from build123d import *

# Parameters (mm, degrees)
EXTRUDE_1_DEPTH     = 4
SKETCH_2_R          = 1.5
CUT_EXTRUDE_1_DEPTH = 53.719070053
CUT_EXTRUDE_3_DEPTH = 2.4
EXTRUDE_2_DEPTH     = 2
FILLET_3_R          = 2
CHAMFER_1_SIZE      = 2


with BuildPart() as part:
    # Эскиз1 → Бобышка-Вытянуть1 (new body)
    with BuildSketch(Plane(origin=(0, 0, 0), x_dir=(0, 0, -1), z_dir=(1, 0, 0))):
        Polygon((-49.583333333, 6.541666667), (-49.583333333, -17.458333333), (-5.983333333, -17.458333333), (-5.983333333, 6.541666667), (-14.983333333, 6.541666667), (-14.983333333, -8.458333333), (-40.583333333, -8.458333333), (-40.583333333, 6.541666667), align=None)
    extrude(amount=EXTRUDE_1_DEPTH)

    # Эскиз2 → Вырез-Вытянуть1 (cut, through all)
    with BuildSketch(Plane.ZY):
        with Locations((10.483333333, 2.190961295)):
            Circle(SKETCH_2_R)
        with Locations((45.083333333, 2.190961295)):
            Circle(SKETCH_2_R)
    extrude(amount=-CUT_EXTRUDE_1_DEPTH, mode=Mode.SUBTRACT)

    # Эскиз4 → Вырез-Вытянуть3 (cut)
    with BuildSketch(Plane.ZY):
        Polygon((10.483333333, 5.337520262), (7.758333333, 3.764240779), (7.758333333, 0.617681812), (10.483333333, -0.955597672), (13.208333333, 0.617681812), (13.208333333, 3.764240779), align=None)
        Polygon((45.083333333, 5.337520262), (42.358333333, 3.764240779), (42.358333333, 0.617681812), (45.083333333, -0.955597672), (47.808333333, 0.617681812), (47.808333333, 3.764240779), align=None)
    extrude(amount=-CUT_EXTRUDE_3_DEPTH, mode=Mode.SUBTRACT)

    # Эскиз6 → Бобышка-Вытянуть2 (add)
    with BuildSketch(Plane.ZY):
        Polygon((5.983333333, -6.458333333), (14.983333333, -6.458333333), (14.983333333, -8.458333333), (40.583333333, -8.458333333), (40.583333333, -6.458333333), (49.583333333, -6.458333333), (49.583333333, -17.458333333), (5.983333333, -17.458333333), align=None)
    extrude(amount=EXTRUDE_2_DEPTH)

    # Скругление3
    fillet_3_edges = [part.edges().sort_by_distance(p)[0] for p in [
        (2, 6.541666667, 40.583333333),
        (2, 6.541666667, 14.983333333),
        (2, 6.541666667, 5.983333333),
        (1, -17.458333333, 5.983333333),
        (1, -17.458333333, 49.583333333),
        (2, 6.541666667, 49.583333333),
    ]]
    fillet(fillet_3_edges, radius=FILLET_3_R)

    # Фаска1
    chamfer_1_edges = [part.edges().sort_by_distance(p)[0] for p in [
        (-2, -6.458333333, 10.483333333),
        (-2, -6.458333333, 45.083333333),
    ]]
    chamfer(chamfer_1_edges, length=CHAMFER_1_SIZE - 0.0001)  # a hair under: the kernel refuses the full size


solid = part.part
For this review, take the finished solid that the model builds, in its own axes (mm). A direction names the side the tool comes from. Give positions to 0.01 mm unless a question says otherwise; leave off trailing zeros. Order: outer loops, then holes, each group sorted by start corner. A loop starts at its lowest first (then second) coordinate and runs counter-clockwise, first axis right, second up. Notation, with made-up numbers: (88, 79) - (100, 79) arc R32 ccw to (100, 118) - close; hole circle Ø5 at (-34, 39.5). An arc over 180 degrees is marked (long way). Answer as a JSON object with one key per item and string values. Group by question number.
Item 1: Wall thickness on line 1 along Z through (x, y) = (1.5, 1.75); line 2 along Z through (x, y) = (2, -4.75); line 3 along Y through (x, z) = (3.25, 26.5): over which ranges is each line inside the solid? List them lowest first.
Item 2: Take a section at B-B on y = 2.75. Give the boundary of the cut face in (x, z), and give its area (3 significant figures).
Item 3: Take a section at C-C on x = 3.5. Give the boundary of the cut face in (y, z), and give its area (3 significant figures).
Item 4: Machinability: for faces 1 (the cylindrical face through (3.189, 2.642, 11.914)), 2 (the cylindrical face through (2.028, 5.971, 41.185)), 3 (the flat face through (2.4, 4, 44)), which of the approach directions +Z, -Z, +X, -X, +Y, -Y give a long, thin tool a straight path to every point of the face, cutting with its end or side? Answer none if there is none.
Item 5: Clearance check with flat-ended pins moving along their axes: pin 1 Ø3 at (y, z) = (-6.5, 40.5) entering from -X; pin 2 Ø4.5 at (y, z) = (1, 10.5) entering from -X; pin 3 Ø3.5 at (y, z) = (2.19, 10.48) entering from -X. State where each tip first meets the part, or that it passes through.
Item 6: Draft analysis for pull direction Z (two halves, no side actions). For faces 4 (the flat face through (1, 2, 42.358)), 5 (the cylindrical face through (2.028, 5.971, 48.982)), 6 (the flat face through (0, -1, 11)), 7 (the cylindrical face through (2.028, 5.971, 6.585)), state which applies: pulls with the +Z half, pulls with the -Z half, needs draft (parallel to the pull), parting line crosses it, or undercut.
Item 7: Take a section at A-A on y = -2.25. Give the boundary of the cut face in (x, z).
Reported:
{
 "1": {"line 1": "5.98 to 7.76, 13.21 to 14.98, 40.58 to 42.36, 47.81 to 49.58", "line 2": "5.98 to 14.98, 40.58 to 49.58", "line 3": "-17.46 to -8.46"},
 "2": {"outline": "(0, 5.98) - (4, 5.98) - (4, 9.09) - (2.4, 9.09) - (2.4, 7.76) - (0, 7.76) - close; (0, 13.21) - (2.4, 13.21) - (2.4, 11.88) - (4, 11.88) - (4, 14.98) - (0, 14.98) - close; (0, 40.58) - (4, 40.58) - (4, 43.69) - (2.4, 43.69) - (2.4, 42.36) - (0, 42.36) - close; (0, 47.81) - (2.4, 47.81) - (2.4, 46.48) - (4, 46.48) - (4, 49.58) - (0, 49.58) - close", "area": "36.9 mm^2"},
 "3": {"outline": "(-17.46, 7.98) arc R2 ccw to (-15.46, 5.98) - (4.54, 5.98) arc R2 ccw to (6.54, 7.98) - (6.54, 12.98) arc R2 ccw to (4.54, 14.98) - (-8.46, 14.98) - (-8.46, 40.58) - (4.54, 40.58) arc R2 ccw to (6.54, 42.58) - (6.54, 47.58) arc R2 ccw to (4.54, 49.58) - (-15.46, 49.58) arc R2 ccw to (-17.46, 47.58) - close; hole circle Ø3 at (2.19, 10.48); hole circle Ø3 at (2.19, 45.08)", "area": "643 mm^2"},
 "4": {"face 1": "+X, -X", "face 2": "+X, -X, +Y", "face 3": "-X"},
 "5": {"pin 1": "x = -1.54", "pin 2": "x = 0", "pin 3": "x = 2.4"},
 "6": {"face 4": "undercut", "face 5": "pulls with the +Z half", "face 6": "needs draft", "face 7": "pulls with the -Z half"},
 "7": {"outline": "(0, 5.98) - (4, 5.98) - (4, 14.98) - (0, 14.98) - close; (0, 40.58) - (4, 40.58) - (4, 49.58) - (0, 49.58) - close"}
}
